from build123d import *

# Parameters (mm, degrees)
SKETCH1_R           = 73.825
SKETCH1_R_2         = 1.65
SKETCH1_R_3         = 1.4
BOSS_EXTRUDE1_DEPTH = 2.5
FILLET1_R           = 4
SKETCH2_R           = 5
SKETCH2_R_2         = 2.75
BOSS_EXTRUDE2_DEPTH = 23.5


with BuildPart() as part:
    # Sketch1 → Boss-Extrude1 (new body)
    with BuildSketch(Plane.XY):
        Circle(SKETCH1_R)
        with Locations((0, 68.825)):
            Circle(SKETCH1_R_2, mode=Mode.SUBTRACT)
        with Locations((68.825, 0)):
            Circle(SKETCH1_R_2, mode=Mode.SUBTRACT)
        with Locations((0, -68.825)):
            Circle(SKETCH1_R_2, mode=Mode.SUBTRACT)
        with Locations((-68.825, 0)):
            Circle(SKETCH1_R_2, mode=Mode.SUBTRACT)
        with Locations((-4.595036818, -58.824966678)):
            Circle(SKETCH1_R_3, mode=Mode.SUBTRACT)
        with Locations((-47.451402468, -35.069295286)):
            Circle(SKETCH1_R_3, mode=Mode.SUBTRACT)
        with Locations((-19.332444494, 15.658647728)):
            Circle(SKETCH1_R_3, mode=Mode.SUBTRACT)
        with Locations((23.523921156, -8.097023664)):
            Circle(SKETCH1_R_3, mode=Mode.SUBTRACT)
        with BuildLine():
            Line((-0.065219366, 63.824966678), (-54.161202477, -33.766770223))
            ThreePointArc((-54.161202477, -33.766770223), (-55.822602808, 30.942974012), (-0.065219366, 63.824966678))
        make_face(mode=Mode.SUBTRACT)
        with BuildLine():
            Line((0.065219366, -63.824966678), (54.161202477, 33.766770223))
            ThreePointArc((54.161202477, 33.766770223), (55.822602808, -30.942974012), (0.065219366, -63.824966678))
        make_face(mode=Mode.SUBTRACT)
        Polygon((-45.430097338, -44.830089012), (13.943787881, 62.283235341), (45.430097338, 44.830089012), (-13.943787881, -62.283235341), align=None, mode=Mode.SUBTRACT)
    extrude(amount=BOSS_EXTRUDE1_DEPTH)

    # Fillet1
    fillet1_edges = [part.edges().sort_by_distance(p)[0] for p in [
        (-0.065219366, 63.824966678, 1.25),
        (-54.161202477, -33.766770223, 1.25),
        (-45.430097338, -44.830089012, 1.25),
        (-13.943787881, -62.283235341, 1.25),
        (45.430097338, 44.830089012, 1.25),
        (13.943787881, 62.283235341, 1.25),
        (54.161202477, 33.766770223, 1.25),
        (0.065219366, -63.824966678, 1.25),
    ]]
    fillet(fillet1_edges, radius=FILLET1_R)

    # Sketch2 → Boss-Extrude2 (add)
    # profile 1 of 2: a face of its own
    with BuildSketch(Plane.XY.offset(2.5)):
        with Locations(Location((-68.825, 0, 0), (0, 0, 179.99962476))):
            Circle(SKETCH2_R)
        with Locations((-68.825, 0)):
            Circle(SKETCH2_R_2, mode=Mode.SUBTRACT)
    # profile 2 of 2: a face of its own
    with BuildSketch(Plane.XY.offset(2.5)):
        with Locations(Location((68.825, 0, 0), (0, 0, 179.999650978))):
            Circle(SKETCH2_R)
        with Locations((68.825, 0)):
            Circle(SKETCH2_R_2, mode=Mode.SUBTRACT)
    extrude(amount=BOSS_EXTRUDE2_DEPTH)


solid = part.part
Geometry: final body of the model. Coordinates: model frame, mm. A direction names the side the tool comes from. Round coordinates to 2 decimals unless told otherwise and drop trailing zeros. Order: outer loops, then holes, each group sorted by start corner. A loop starts at its lowest first (then second) coordinate and runs counter-clockwise, first axis right, second up. Notation, with made-up numbers: (20.25, 66) - (52.25, 66) arc R16 ccw to (52.25, 84) - close; hole circle Ø4 at (-18, -19). An arc over 180 degrees is marked (long way). Write each question's results on one line, items separated by ' | '.
Item 1: Section B-B, the plane x = -54.5. Return the cut outline in (y, z).
Completed:
outline: (-49.8, 0) - (-29.45, 0) - (-29.45, 2.5) - (-49.8, 2.5) - close; (33.22, 0) - (49.8, 0) - (49.8, 2.5) - (33.22, 2.5) - close
Item 2: Mould query, pull axis X, two halves, no side actions, for faces 4 (the flat face through (66.7, 2.2, 26)), 5 (the cylindrical face through (-9.6, 73.2, 1.2)), 6 (the cylindrical face through (66.078, 0.121, 14.086)). Classes: pulls with the +X half, pulls with the -X half, needs draft (parallel to the pull), parting line crosses it, or undercut.
Completed:
face 4: needs draft | face 5: parting line crosses it | face 6: undercut
Item 3: Material intervals for line 1 along Y through (x, z) = (0, 1) (3 decimals); line 2 along X through (y, z) = (-23, 2); line 3 along X through (y, z) = (-0.5, 24.5), sorted ascending. Write a range as [from, to].
Completed:
line 1: [-73.825, -70.475], [-67.175, -37.128], [37.128, 67.175], [70.475, 73.825] | line 2: [-70.15, -59.54], [-48.19, -33.33], [7.83, 22.69], [59.54, 70.15] | line 3: [-73.8, -71.53], [-66.12, -63.85], [63.85, 66.12], [71.53, 73.8]
Item 4: Section A-A, the plane y = -54. Return the cut outline in (x, z), and give its area (3 significant figures).
Completed:
outline: (-50.34, 0) - (-28.89, 0) - (-28.89, 2.5) - (-50.34, 2.5) - close; (-9.35, 0) - (5.51, 0) - (5.51, 2.5) - (-9.35, 2.5) - close; (34.02, 0) - (50.34, 0) - (50.34, 2.5) - (34.02, 2.5) - close | area: 132 mm^2
Item 5: Reachability of faces 1 (the cylindrical face through (-73.44, 1.92, 14.09)), 2 (the flat face through (26.784, -15.623, 1.232)), 3 (the flat face through (-71, 2, 26)) from +Z, -Z, +X, -X, +Y, -Y: full face, straight path, thin tool, end or side. Return the list, or none.
Completed:
face 1: +Z | face 2: +Z, -Z | face 3: +Z, +X, -X, +Y, -Y
Item 6: Section D-D, the plane z = 23. Return the cut outline in (x, y) (3 decimals).
Completed:
outline: circle Ø10 at (-68.825, 0); circle Ø10 at (68.825, 0); hole circle Ø5.5 at (-68.825, 0); hole circle Ø5.5 at (68.825, 0)
Item 7: Section C-C, the plane y = -21. Return the cut outline in (x, z), and give its area (3 significant figures).
Completed:
outline: (-70.78, 0) - (-60.27, 0) - (-60.27, 2.5) - (-70.78, 2.5) - close; (-47.08, 0) - (-32.22, 0) - (-32.22, 2.5) - (-47.08, 2.5) - close; (8.94, 0) - (23.8, 0) - (23.8, 2.5) - (8.94, 2.5) - close; (60.27, 0) - (70.78, 0) - (70.78, 2.5) - (60.27, 2.5) - close | area: 127 mm^2
Item 8: First-contact query: pin 1 Ø8 at (x, z) = (3, 10) entering from -Y; pin 2 Ø1.6 at (x, y) = (-69, -1) entering from +Z; pin 3 Ø12 at (x, z) = (-11.5, 4.5) entering from +Y; pin 4 Ø9 at (x, y) = (68.825, 0) entering from -Z. Flat tips, straight axial feed; report the tip coordinate or a pass-through.
Completed:
pin 1: through | pin 2: z = 2.5 | pin 3: y = 73.59 | pin 4: z = 0
